from build123d import *

# Parameters (mm, degrees)
SKETCH_1_R         = 11
SKETCH_1_R_2       = 1.55
SKETCH_1_R_3       = 19
EXTRUDE_1_DEPTH    = 7
SKETCH1_R          = 2.75
CUT_EXTRUDE1_DEPTH = 3
SKETCH2_R          = 12.025
CUT_EXTRUDE2_DEPTH = 5


with BuildPart() as part:
    # 草图1 → 凸台-拉伸1 (new body)
    # profile 1 of 3: a face of its own
    with BuildSketch(Plane.XY):
        with BuildLine():
            ThreePointArc((19, 80), (0, 99), (-19, 80))
            ThreePointArc((-19, 80), (0, 61), (19, 80))
        make_face()
        with Locations((0, 80)):
            Circle(SKETCH_1_R, mode=Mode.SUBTRACT)
    # profile 2 of 3: a face of its own
    with BuildSketch(Plane.XY):
        with BuildLine():
            Line((-19, 7), (-19, 0))
            Line((-19, 0), (19, 0))
            Line((19, 0), (19, 7))
            Line((19, 7), (19, 80))
            ThreePointArc((19, 80), (0, 61), (-19, 80))
            Line((-19, 80), (-19, 7))
        make_face()
        with Locations((-15, 3.5)):
            Circle(SKETCH_1_R_2, mode=Mode.SUBTRACT)
        with BuildLine():
            ThreePointArc((-7.5, 45), (0, 52.5), (7.5, 45))
            Line((7.5, 45), (7.5, 15))
            ThreePointArc((7.5, 15), (0, 7.5), (-7.5, 15))
            Line((-7.5, 15), (-7.5, 45))
        make_face(mode=Mode.SUBTRACT)
        with Locations((15, 3.5)):
            Circle(SKETCH_1_R_2, mode=Mode.SUBTRACT)
    # profile 3 of 3: a face of its own
    with BuildSketch(Plane.XY):
        with Locations((0, 80)):
            Circle(SKETCH_1_R_3)
        with Locations((0, 80)):
            Circle(SKETCH_1_R, mode=Mode.SUBTRACT)
    extrude(amount=EXTRUDE_1_DEPTH)

    # Sketch1 → Cut-Extrude1 (cut)
    with BuildSketch(Plane.XY.offset(7)):
        with Locations((15, 3.5)):
            Circle(SKETCH1_R)
        with Locations(Location((-15, 3.5, 0), (0, 0, 180))):
            Circle(SKETCH1_R)
    extrude(amount=-CUT_EXTRUDE1_DEPTH, mode=Mode.SUBTRACT)

    # Sketch2 → Cut-Extrude2 (cut)
    with BuildSketch(Plane(origin=(0, 0, 0), x_dir=(-1, 0, 0), z_dir=(0, 0, -1))):
        with Locations((0, 80)):
            Circle(SKETCH2_R)
    extrude(amount=-CUT_EXTRUDE2_DEPTH, mode=Mode.SUBTRACT)


solid = part.part
Can you work these out from the model? Positions are in its coordinate system, mm. A direction names the side the tool comes from. Coordinates: 2 decimals unless noted, no trailing zeros. Write each loop counter-clockwise with the first axis right and the second up, starting at its lowest first coordinate (ties: lowest second). Pieces come first, ordered by that corner, then holes.
Q1. Imagine slicing it at C-C, the plane y = 3.5. List the corners of the cut face in (x, z) for me, plus the area to 3 significant figures.
Results found:
outline: (-19, 0) - (-16.55, 0) - (-16.55, 4) - (-17.75, 4) - (-17.75, 7) - (-19, 7) - close; (-13.45, 0) - (13.45, 0) - (13.45, 4) - (12.25, 4) - (12.25, 7) - (-12.25, 7) - (-12.25, 4) - (-13.45, 4) - close; (16.55, 0) - (19, 0) - (19, 7) - (17.75, 7) - (17.75, 4) - (16.55, 4) - close
area: 208 mm2
Q2. Imagine slicing it at B-B, the plane z = 6. List the corners of the cut face in (x, y) for me, plus the area to 3 significant figures.
Results found:
outline: (-19, 0) - (19, 0) - (19, 80) arc R19 ccw to (-19, 80) - close; hole circle Ø5.5 at (-15, 3.5); hole circle Ø22 at (0, 80); hole (-7.5, 15) arc R7.5 ccw to (7.5, 15) - (7.5, 45) arc R7.5 ccw to (-7.5, 45) - close; hole circle Ø5.5 at (15, 3.5)
area: 2,550 mm2
Q3. Which directions (+Z, -Z, +X, -X, +Y, -Y) give clear straight access to the entire face, cutting with the end or side of a thin tool? Please do faces 5 (the face through (-7.5, 30, 3)), 6 (the face through (8, 50, 0)), 7 (the face through (-10, 75, 5)), 8 (the face through (0, 99, 3)), 9 (the face through (-16, 5, 4)).
Results found:
face 5: +Z, -Z
face 6: -Z, +X, -X, +Y, -Y
face 7: -Z
face 8: +Z, -Z, +Y
face 9: +Z
Q4. For P1, Ø13, axis at x = 0, y = 80, coming from the +Z side, with a flat end and sliding along its axis, tell me the tip position at first contact or that it passes through.
Results found:
P1: passes through
Q5. Imagine slicing it at D-D, the plane x = 15. List the corners of the cut face in (y, z) for me.
Results found:
outline: (0, 0) - (1.95, 0) - (1.95, 4) - (0.75, 4) - (0.75, 7) - (0, 7) - close; (5.05, 0) - (91.66, 0) - (91.66, 7) - (6.25, 7) - (6.25, 4) - (5.05, 4) - close
Q6. Imagine slicing it at A-A, the plane x = 0. List the corners of the cut face in (y, z) for me (3 decimals).
Results found:
outline: (0, 0) - (7.5, 0) - (7.5, 7) - (0, 7) - close; (52.5, 0) - (67.975, 0) - (67.975, 5) - (69, 5) - (69, 7) - (52.5, 7) - close; (91, 5) - (92.025, 5) - (92.025, 0) - (99, 0) - (99, 7) - (91, 7) - close
Q7. Please list where these lines run through material, in increasing order: L1, parallel to Y at x = 0, z = 2.65 (3 decimals); L2, parallel to X at y = 3.5, z = 2.5; L3, parallel to Y at x = 1, z = 5.75.
Results found:
L1: y = 0 to 7.5, 52.5 to 67.975, 92.025 to 99
L2: x = -19 to -16.55, -13.45 to 13.45, 16.55 to 19
L3: y = 0 to 7.57, 52.43 to 69.05, 90.95 to 98.97
Q8. If we mould it in two halves opening along X, with no side actions, what happens to faces 1 (the face through (19, 39, 3)), 2 (the face through (-16.55, 3.57, 1.97)), 3 (the face through (-19, 41, 3)), 4 (the face through (0, 0, 3))? For each: +X half, -X half, draft (parallel to the pull), parting line (faces both ways), or undercut.
Results found:
face 1: +X half
face 2: undercut
face 3: -X half
face 4: draft
